from build123d import *

# Parameters (mm, degrees)
BLOCK_DEPTH                           = 25.25
TAP_DRILL_FOR_M5X0_8_TAP1_D           = 4.2
TAP_DRILL_FOR_M5X0_8_TAP1_DEPTH       = 7.5
TAP_DRILL_FOR_M5X0_8_TAP1_CSINK_D     = 4.25
TAP_DRILL_FOR_M5X0_8_TAP1_CSINK_ANGLE = 90
TAP_DRILL_FOR_M5X0_8_TAP1_TIP         = 1.093190806
F_6_0_6_DIAMETER_HOLE1_D              = 6


with BuildPart() as part:
    # Sketch2 → Block (new, symmetric)
    with BuildSketch(Plane.XY):
        with BuildLine():
            Line((-7.230720611, 12.9), (7.230720611, 12.9))
            Line((7.230720611, 12.9), (7.647672674, 12.483047938))
            ThreePointArc((7.647672674, 12.483047938), (7.736182466, 12.363118479), (7.785406885, 12.222427275))
            ThreePointArc((7.785406885, 12.222427275), (8.344607784, 11.164307384), (9.402727675, 10.605106485))
            ThreePointArc((9.402727675, 10.605106485), (9.54341888, 10.555882066), (9.663348338, 10.467372274))
            Line((9.663348338, 10.467372274), (9.853553391, 10.277167221))
            ThreePointArc((9.853553391, 10.277167221), (9.961939766, 10.114955546), (10, 9.92361383))
            Line((10, 9.92361383), (10, 8.86638617))
            ThreePointArc((10, 8.86638617), (9.961939766, 8.675044454), (9.853553391, 8.512832779))
            Line((9.853553391, 8.512832779), (9.675343394, 8.334622782))
            ThreePointArc((9.675343394, 8.334622782), (9.554347216, 8.245550888), (9.412352167, 8.19644607))
            ThreePointArc((9.412352167, 8.19644607), (8.344607784, 7.635448616), (7.783610331, 6.567704234))
            ThreePointArc((7.783610331, 6.567704234), (7.734505512, 6.425709184), (7.645433618, 6.304713007))
            Line((7.645433618, 6.304713007), (6.892893219, 5.552172608))
            ThreePointArc((6.892893219, 5.552172608), (6.676120468, 5.227749259), (6.6, 4.845065826))
            Line((6.6, 4.845065826), (6.6, 3.284934173))
            ThreePointArc((6.6, 3.284934173), (6.676120468, 2.902250741), (6.892893219, 2.577827392))
            Line((6.892893219, 2.577827392), (9.470720611, 0))
            Line((9.470720611, 0), (19.9998779, 0))
            Line((19.9998779, 0), (21.5001221, 1.5))
            Line((21.5001221, 1.5), (21.5001221, 11.9))
            Line((21.5001221, 11.9), (22, 12.3997558))
            Line((22, 12.3997558), (22, 24.4))
            Line((22, 24.4), (20.9998779, 25.4))
            Line((20.9998779, 25.4), (11.9998779, 25.4))
            Line((11.9998779, 25.4), (11.792771119, 25.192893219))
            ThreePointArc((11.792771119, 25.192893219), (11.46834777, 24.976120467), (11.085664338, 24.9))
            Line((11.085664338, 24.9), (4.914091462, 24.9))
            ThreePointArc((4.914091462, 24.9), (4.53140803, 24.976120467), (4.206984681, 25.192893219))
            Line((4.206984681, 25.192893219), (4.0001221, 25.4))
            Line((4.0001221, 25.4), (-3.9998779, 25.4))
            Line((-3.9998779, 25.4), (-4.206984681, 25.192893219))
            ThreePointArc((-4.206984681, 25.192893219), (-4.53140803, 24.976120467), (-4.914091462, 24.9))
            Line((-4.914091462, 24.9), (-11.085664338, 24.9))
            ThreePointArc((-11.085664338, 24.9), (-11.46834777, 24.976120467), (-11.792771119, 25.192893219))
            Line((-11.792771119, 25.192893219), (-11.9998779, 25.4))
            Line((-11.9998779, 25.4), (-20.9998779, 25.4))
            Line((-20.9998779, 25.4), (-22, 24.4))
            Line((-22, 24.4), (-22, 17.4))
            Line((-22, 17.4), (-21.5001221, 16.9002442))
            Line((-21.5001221, 16.9002442), (-21.5001221, 1.5))
            Line((-21.5001221, 1.5), (-19.9998779, 0))
            Line((-19.9998779, 0), (-9.470720611, 0))
            Line((-9.470720611, 0), (-6.892893219, 2.577827392))
            ThreePointArc((-6.892893219, 2.577827392), (-6.676120468, 2.902250741), (-6.6, 3.284934173))
            Line((-6.6, 3.284934173), (-6.6, 4.845065826))
            ThreePointArc((-6.6, 4.845065826), (-6.676120468, 5.227749259), (-6.892893219, 5.552172608))
            Line((-6.892893219, 5.552172608), (-7.645433618, 6.304713006))
            ThreePointArc((-7.645433618, 6.304713006), (-7.734505512, 6.425709184), (-7.783610331, 6.567704233))
            ThreePointArc((-7.783610331, 6.567704233), (-8.344607784, 7.635448616), (-9.412352167, 8.19644607))
            ThreePointArc((-9.412352167, 8.19644607), (-9.554347216, 8.245550888), (-9.675343394, 8.334622782))
            Line((-9.675343394, 8.334622782), (-9.853553391, 8.512832779))
            ThreePointArc((-9.853553391, 8.512832779), (-9.961939766, 8.675044454), (-10, 8.86638617))
            Line((-10, 8.86638617), (-10, 9.92361383))
            ThreePointArc((-10, 9.92361383), (-9.961939766, 10.114955546), (-9.853553391, 10.277167221))
            Line((-9.853553391, 10.277167221), (-9.663348338, 10.467372274))
            ThreePointArc((-9.663348338, 10.467372274), (-9.543418879, 10.555882066), (-9.402727675, 10.605106485))
            ThreePointArc((-9.402727675, 10.605106485), (-8.344607784, 11.164307384), (-7.785406885, 12.222427275))
            ThreePointArc((-7.785406885, 12.222427275), (-7.736182466, 12.363118479), (-7.647672674, 12.483047938))
            Line((-7.647672674, 12.483047938), (-7.230720611, 12.9))
        make_face()
    extrude(amount=BLOCK_DEPTH, both=True)

    # Tap Drill for M5x0.8 Tap1
    with Locations(Plane(origin=(0, 25.4, 0), x_dir=(1, 0, 0), z_dir=(0, 1, 0))):
        with Locations((16, 18), (-16, 18), (16, -18), (-16, -18)):
            CounterSinkHole(TAP_DRILL_FOR_M5X0_8_TAP1_D / 2, TAP_DRILL_FOR_M5X0_8_TAP1_CSINK_D / 2, depth=TAP_DRILL_FOR_M5X0_8_TAP1_DEPTH, counter_sink_angle=TAP_DRILL_FOR_M5X0_8_TAP1_CSINK_ANGLE)
            with Locations((0, 0, -(TAP_DRILL_FOR_M5X0_8_TAP1_DEPTH + TAP_DRILL_FOR_M5X0_8_TAP1_TIP / 2))):  # 125° drill point
                Cone(0, TAP_DRILL_FOR_M5X0_8_TAP1_D / 2, TAP_DRILL_FOR_M5X0_8_TAP1_TIP, mode=Mode.SUBTRACT)

    # Ø6.0 (6) Diameter Hole1 (through all)
    with Locations(Plane(origin=(0, 0, -25.25), x_dir=(-1, 0, 0), z_dir=(0, 0, -1))):
        with Locations((0, 19.4)):
            Hole(F_6_0_6_DIAMETER_HOLE1_D / 2)


solid = part.part
Source: CAD feature listing. Evaluate the final solid. Frame: model axes, mm. A direction names the side the tool comes from. Give positions to 0.01 mm unless a question says otherwise; leave off trailing zeros. Write each loop counter-clockwise with the first axis right and the second up, starting at its lowest first coordinate (ties: lowest second). Pieces come first, ordered by that corner, then holes. Notation, with made-up numbers: (-19.75, -23) -> (17.25, -23) arc R18 ccw to (17.25, 7) -> close; hole circle Ø8 at (55.25, 56). An arc over 180 degrees is marked (long way). Return JSON: item names as keys, results as strings. Group by question number.
1. Access query for faces 4 (the face through (-21.5, 9, 0)), 5 (the face through (-8.33, 7.62, 0.35)), 6 (the face through (-8.2, 1.27, 0.35)), 7 (the face through (14.87, 21.59, -19.77)). Directions: +Z, -Z, +X, -X, +Y, -Y. A direction counts if a zero-diameter tool reaches every point of the face in a straight line with its end or side. Return the directions, or none.
2. Section A-A, the plane y = 23.75. Output: boundary loops of the cut face in (x, z).
3. Pin query (flat end, axial travel): pin 1 Ø0.8 at (y, z) = (4, -2) entering from -X; pin 2 Ø1.2 at (y, z) = (9.5, 4.5) entering from +X; pin 3 Ø3.5 at (x, z) = (16, -18) entering from +Y. Return the tip coordinate at first contact, or that it passes through.
4. Mould query, pull axis Z, two halves, no side actions, for faces 1 (the face through (0, 16, 25.25)), 2 (the face through (-16.097, 16.875, 17.911)), 3 (the face through (8, 24.9, 0)). Classes: +Z half, -Z half, draft (parallel to the pull), parting line (faces both ways), or undercut.
5. Material intervals for line 1 (Z direction, x = -16, y = 21.5); line 2 (X direction, y = 23.75, z = -18); line 3 (X direction, y = 9, z = -22), sorted ascending. Write a range as from..to.
Determined:
{
 "1": {"face 4": "+Z, -Z, -X, -Y", "face 5": "+Z, -Z", "face 6": "+Z, -Z, -Y", "face 7": "+Y"},
 "2": {"outline": "(-22, -25.25) -> (22, -25.25) -> (22, 25.25) -> (-22, 25.25) -> close; hole circle Ø4.2 at (-16, -18); hole circle Ø4.2 at (-16, 18); hole circle Ø4.2 at (16, -18); hole circle Ø4.2 at (16, 18)"},
 "3": {"pin 1": "stops at x = -21.5", "pin 2": "stops at x = 21.5", "pin 3": "stops at y = 17.72"},
 "4": {"face 1": "+Z half", "face 2": "undercut", "face 3": "draft"},
 "5": {"line 1": "z = -25.25..-20.1, -15.9..15.9, 20.1..25.25", "line 2": "x = -22..-18.1, -13.9..13.9, 18.1..22", "line 3": "x = -21.5..-10, 10..21.5"}
}
